```python
from build123d import *

# Parameters (mm, degrees)
SKETCH2_R               = 12
SKETCH2_R_2             = 8
BOSS_EXTRUDE1_DEPTH     = 8
CUT_EXTRUDE1_DEPTH      = 19.761663039
CUT_EXTRUDE1_DEPTH_BACK = 19.761663039
SKETCH3_R               = 2
CHAMFER1_SIZE           = 1


with BuildPart() as part:
    # Sketch2 → Boss-Extrude1 (new body)
    with BuildSketch(Plane(origin=(0, 0, 0), x_dir=(1, 0, 0), z_dir=(0, 1, 0))):
        with Locations(Location((0, 0, 0), (0, 0, 270))):
            Circle(SKETCH2_R)
        with Locations(Location((0, 0, 0), (0, 0, 270))):
            Circle(SKETCH2_R_2, mode=Mode.SUBTRACT)
    extrude(amount=BOSS_EXTRUDE1_DEPTH)

    # Sketch3 → Cut-Extrude1 (cut, two sides: drawn at the far end of the back side and taken through both)
    with BuildSketch(Plane.XY.offset(-CUT_EXTRUDE1_DEPTH_BACK)):
        with Locations((0, 4)):
            Circle(SKETCH3_R)
    extrude(amount=CUT_EXTRUDE1_DEPTH + CUT_EXTRUDE1_DEPTH_BACK, mode=Mode.SUBTRACT)

    # Chamfer1
    chamfer1_edges = [part.edges().sort_by_distance(p)[0] for p in [
        (0, 8, -12),
    ]]
    chamfer(chamfer1_edges, length=CHAMFER1_SIZE)


solid = part.part
```
Here's how the part is built. I have some questions about the finished solid (model axes, mm). Give positions to 0.01 mm unless a question says otherwise; leave off trailing zeros. Order: outer loops, then holes, each group sorted by start corner. A loop starts at its lowest first (then second) coordinate and runs counter-clockwise, first axis right, second up. Notation, with made-up numbers: M 43,74 L 72,74 A30 cw 72,110 Z; hole C 67.25,0.25 d10. An arc over 180 degrees is marked long. Use a Markdown table: item, result. Add a question column.
1. Suppose I cut it at B-B (z = 0). List the corners of the cut face in (x, y) for me, and give its area (3 significant figures).
2. Suppose I cut it at D-D (y = 4.75). List the corners of the cut face in (x, z) for me.
3. Suppose I cut it at C-C (y = 3). List the corners of the cut face in (x, z) for me.
4. I need wall thicknesses on probe 1 along Y at (x, z) = (0, 9.9); probe 2 along X at (y, z) = (5, 0); probe 3 along X at (y, z) = (5.25, -6.5). Which ranges of each line are inside material? Lowest first, please. Write a range as from..to.
5. If we mould it in two halves opening along X, with no side actions, what happens to faces 1 (the cylindrical face through (3.604, 3.451, 11.446)), 2 (the flat face through (-8, 8, -2)), 3 (the cylindrical face through (-3.06, 3.94, 7.39))? For each: +X half, -X half, draft (parallel to the pull), parting line (faces both ways), or undercut.
6. Suppose I cut it at A-A (x = 0). List the corners of the cut face in (y, z) for me.
7. For pin 1 Ø2.5 at (x, y) = (0, 4) entering from +Z; pin 2 Ø8 at (x, z) = (-9, 0) entering from -Y; pin 3 Ø4 at (x, y) = (-7, 2) entering from +Z; pin 4 Ø1.5 at (y, z) = (2, 9) entering from +X, each with a flat end and sliding along its axis, tell me the tip position at first contact or that it passes through.
Results list:
| question | item | result |
|---|---|---|
| 1 | outline | M -12,0 L -8,0 L -8,8 L -11,8 L -12,7 Z; M 8,0 L 12,0 L 12,7 L 11,8 L 8,8 Z |
| 1 | area | 63.0 mm² |
| 2 | outline | M -1.85,-11.86 L -1.85,-7.78 A8 cw -1.85,7.78 L -1.85,11.86 A12 ccw Z; M 1.85,-11.86 A12 ccw 1.85,11.86 L 1.85,7.78 A8 cw 1.85,-7.78 Z |
| 3 | outline | M -1.73,-11.87 L -1.73,-7.81 A8 cw -1.73,7.81 L -1.73,11.87 A12 ccw Z; M 1.73,-11.87 A12 ccw 1.73,11.87 L 1.73,7.81 A8 cw 1.73,-7.81 Z |
| 4 | probe 1 | y = 0..2, 6..8 |
| 4 | probe 2 | x = -12..-8, 8..12 |
| 4 | probe 3 | x = -10.09..-4.66, 4.66..10.09 |
| 5 | face 1 | parting line |
| 5 | face 2 | draft |
| 5 | face 3 | undercut |
| 6 | outline | M 0,-12 L 2,-12 L 2,-8 L 0,-8 Z; M 0,8 L 2,8 L 2,12 L 0,12 Z; M 6,-12 L 7,-12 L 8,-11 L 8,-8 L 6,-8 Z; M 6,8 L 8,8 L 8,11 L 7,12 L 6,12 Z |
| 7 | pin 1 | passes through |
| 7 | pin 2 | stops at y = 0 |
| 7 | pin 3 | stops at z = 10.91 |
| 7 | pin 4 | stops at x = 8.71 |
